from build123d import *

# Parameters (mm, degrees)
F1_DEPTH = 12.7
F2_R     = 4.0005
F3_DEPTH = 12.7


with BuildPart() as f1:
    # F0 (on Front) → F1 (new body)
    with BuildSketch(Plane.XZ):
        with BuildLine():
            ThreePointArc((-39.4, -8.001), (-33.742439, -5.657561), (-31.399, 0))
            ThreePointArc((-31.399, 0), (-33.742439, 5.657561), (-39.4, 8.001))
            ThreePointArc((-39.4, 8.001), (-47.401, 0), (-39.4, -8.001))
        make_face()
        with BuildLine():
            ThreePointArc((-39.4, 8.001), (-33.742439, 5.657561), (-31.399, 0))
            ThreePointArc((-31.399, 0), (-33.742439, -5.657561), (-39.4, -8.001))
            Line((-39.4, -8.001), (0, -8.001))
            ThreePointArc((0, -8.001), (-8.001, 0), (0, 8.001))
            Line((0, 8.001), (-39.4, 8.001))
        make_face()
        with BuildLine():
            ThreePointArc((8.001, 0), (5.657561, 5.657561), (0, 8.001))
            ThreePointArc((0, 8.001), (-8.001, 0), (0, -8.001))
            ThreePointArc((0, -8.001), (5.657561, -5.657561), (8.001, 0))
        make_face()
    extrude(amount=F1_DEPTH)

    # F2 (on face) → F3 (cut, through all)
    with BuildSketch(Plane.XZ.offset(12.7)):
        with Locations((-39.4, 0)):
            Circle(F2_R)
        Circle(F2_R)
    extrude(amount=-F3_DEPTH, mode=Mode.SUBTRACT)


solid = f1.part
For this review, take the finished solid that the model builds, in its own axes (mm). Round coordinates to 2 decimals unless told otherwise and drop trailing zeros. Order: outer loops, then holes, each group sorted by start corner. A loop starts at its lowest first (then second) coordinate and runs counter-clockwise, first axis right, second up. Notation, with made-up numbers: (32.5, -22) -> (78.5, -22) arc R26 ccw to (78.5, -5) -> close; hole circle Ø4 at (1.5, -36). An arc over 180 degrees is marked (long way). Write item = value, one per line. Start each with the question number.
1) Take a section at C-C on z = -0.75. State the section outline as (x, y) points.
2) Insertion check: pin 1 (4 mm diameter, centred on y = -7.5, z = -5, fed in from -X). The pin has a flat end and moves straight along its axis. Give the tip position at first contact, or say it passes through.
3) Take a section at A-A on y = -3.25. State the section outline as (x, z) points, plus the area to 3 significant figures.
4) To check wall thickness, follow line 1 (Z direction, x = 0, y = -4.5); line 2 (X direction, y = -11.5, z = 2.75); line 3 (X direction, y = -6.5, z = 1). State the ranges of each line that lie inside material, in increasing order. Write a range as from..to.
5) Take a section at B-B on x = -0.5. State the section outline as (y, z) points.
6) The part is to be moulded in two halves that separate along X. For faces 1 (the face through (-0.9, -6.4, -3.9)), 2 (the face through (-20, -6, -8.001)), 3 (the face through (-47.4, -6.3, 0.2)), say which applies: +X half, -X half, draft (parallel to the pull), parting line (faces both ways), or undercut.
7) Take a section at D-D on z = -5. State the section outline as (x, y) points.
Verdict:
q1.outline = (-47.37, -12.7) -> (-43.33, -12.7) -> (-43.33, 0) -> (-47.37, 0) -> close; (-35.47, -12.7) -> (-3.93, -12.7) -> (-3.93, 0) -> (-35.47, 0) -> close; (3.93, -12.7) -> (7.97, -12.7) -> (7.97, 0) -> (3.93, 0) -> close
q2.pin_1 = -46.82
q3.outline = (-39.4, -8) -> (0, -8) arc R8 ccw to (8, 0) arc R8 ccw to (0, 8) -> (-39.4, 8) arc R8 ccw to start; hole circle Ø8 at (-39.4, 0); hole circle Ø8 at (0, 0)
q3.area = 731 mm2
q4.line_1 = -8..-4, 4..8
q4.line_2 = -46.91..-42.31, -36.49..-2.91, 2.91..7.51
q4.line_3 = -47.34..-43.27, -35.53..-3.87, 3.87..7.94
q5.outline = (-12.7, -8) -> (0, -8) -> (0, -3.97) -> (-12.7, -3.97) -> close; (-12.7, 3.97) -> (0, 3.97) -> (0, 8) -> (-12.7, 8) -> close
q6.face_1 = undercut
q6.face_2 = draft
q6.face_3 = -X half
q7.outline = (-45.65, -12.7) -> (6.25, -12.7) -> (6.25, 0) -> (-45.65, 0) -> close
